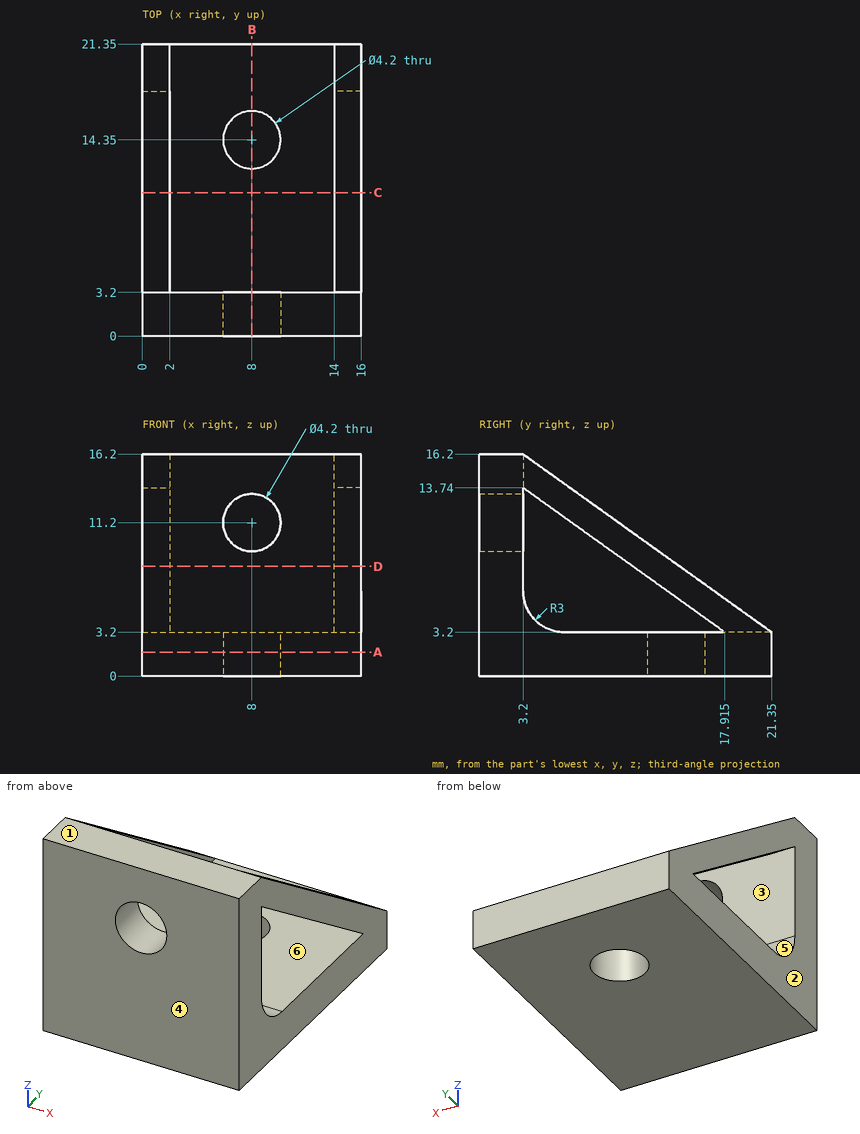
For this review, use the dimensioned drawing (mm, ordinates from the lowest corner) and the shaded views. A direction names the side the tool comes from. Coordinates: 2 decimals unless noted, no trailing zeros. Order: outer loops, then holes, each group sorted by start corner. A loop starts at its lowest first (then second) coordinate and runs counter-clockwise, first axis right, second up. Notation, with made-up numbers: M -24,0.25 L 24,0.25 A22 cw 24,18.25 Z; hole C -19,89 d6. An arc over 180 degrees is marked long. Answer as a JSON object with one key per item and string values. Group by question number.
1) Add section A-A, the plane z = 1.75. Write out the cut boundary in (x, y).
2) Add section D-D, the plane z = 8. Write out the cut boundary in (x, y).
3) Add section B-B, the plane x = 8. Write out the cut boundary in (y, z).
4) Wall thickness on L1, parallel to Y at x = 8, z = 2.3; L2, parallel to X at y = 2.25, z = 11.2; L3, parallel to Z at x = 8, y = 2.45: over which ranges is each line inside the solid? List them lowest first.
5) For pin 1 (3.5 mm diameter, centred on x = 8, z = 11.2, fed in from -Y); pin 2 (3 mm diameter, centred on x = 7.5, z = 12.5, fed in from +Y); pin 3 (8 mm diameter, centred on x = 14, y = 19, fed in from +Z); pin 4 (1 mm diameter, centred on x = 5, y = 16, fed in from +Z), all flat-tipped, find the tip position at first contact; note any pin that passes through.
6) Add section C-C, the plane y = 10.5. Write out the cut boundary in (x, z).
7) Mouldability with a two-part tool opening along X and no side actions: class the marked faces 1, 2 and 3 as pulls with the +X half, pulls with the -X half, needs draft (parallel to the pull), parting line crosses it, or undercut.
8) Tool access review of the marked faces 4, 5 and 6: name each direction out of +Z, -Z, +X, -X, +Y, -Y from which nothing blocks a thin tool from reaching the whole face with its end or side.
Computed values:
{
 "1": {"outline": "M 0,0 L 16,0 L 16,21.35 L 0,21.35 Z; hole C 8,14.35 d4.2"},
 "2": {"outline": "M 0,0 L 16,0 L 16,3.2 L 0,3.2 Z; M 0,11.21 L 2,11.21 L 2,14.65 L 0,14.65 Z; M 14,11.21 L 16,11.21 L 16,14.65 L 14,14.65 Z"},
 "3": {"outline": "M 0,0 L 12.25,0 L 12.25,3.2 L 6.2,3.2 A3 cw 3.2,6.2 L 3.2,9.1 L 0,9.1 Z; M 0,13.3 L 3.2,13.3 L 3.2,16.2 L 0,16.2 Z; M 16.45,0 L 21.35,0 L 21.35,3.2 L 16.45,3.2 Z"},
 "4": {"L1": "y = 0 to 12.25, 16.45 to 21.35", "L2": "x = 0 to 5.9, 10.1 to 16", "L3": "z = 0 to 9.1, 13.3 to 16.2"},
 "5": {"pin 1": "passes through", "pin 2": "stops at y = 3.2", "pin 3": "stops at z = 7.75", "pin 4": "stops at z = 3.2"},
 "6": {"outline": "M 0,0 L 16,0 L 16,3.2 L 0,3.2 Z; M 0,8.51 L 2,8.51 L 2,10.97 L 0,10.97 Z; M 14,8.51 L 16,8.51 L 16,10.97 L 14,10.97 Z"},
 "7": {"face 1": "needs draft", "face 2": "pulls with the -X half", "face 3": "undercut"},
 "8": {"face 4": "+Z, -Z, +X, -X, -Y", "face 5": "+X, -X", "face 6": "none"}
}
